Model file for the job. Use its own axes, mm. A direction names the side the tool comes from. Round coordinates to 2 decimals unless told otherwise and drop trailing zeros. Order: outer loops, then holes, each group sorted by start corner. A loop starts at its lowest first (then second) coordinate and runs counter-clockwise, first axis right, second up. Notation, with made-up numbers: M 25.5,-34 L 48.5,-34 A18 cw 48.5,-20 Z; hole C 55.5,53 d1. An arc over 180 degrees is marked long. Return JSON: item names as keys, results as strings. Group by question number.
Item 1: Pull direction X, two halves, no side cores. Call faces 5 (the face through (-5.5, -2, 0)), 6 (the face through (19, -13, 25)), 7 (the face through (42.5, -2, 0)): pulls with the +X half, pulls with the -X half, needs draft (parallel to the pull), parting line crosses it, or undercut.
Item 2: Slice it at C-C on x = 40.5. Write the cut outline in (y, z), then the cut area to 3 significant figures.
Item 3: Probe line 1 along Y through (x, z) = (50.5, 10); line 2 along X through (y, z) = (7.5, 2.5) (3 decimals); line 3 along Y through (x, z) = (-7, -16.5). List the from-to ranges inside material, lowest first.
Item 4: Slice it at A-A on z = -5. Write the cut outline in (x, y), then the cut area to 3 significant figures.
Item 5: Pin check, flat tips, straight feed: pin 1 Ø8 at (x, z) = (4, -3.5) entering from +Y; pin 2 Ø8 at (x, y) = (-1.5, 6.5) entering from -Z; pin 3 Ø1.5 at (x, z) = (-5, -13) entering from +Y. Stop position of each tip, or through.
Item 6: Slice it at B-B on y = 3. Write the cut outline in (x, z), then the cut area to 3 significant figures.
Item 7: Which spindle directions (+Z, -Z, +X, -X, +Y, -Y) get a long thin tool onto all of the face, cutting with end or side? Do faces 1 (the face through (-2, 0, -10)), 2 (the face through (-15, -19, 0)), 3 (the face through (39, 0, -10)), 4 (the face through (39, 0, 10)). Say none if no direction does.
Item 8: Slice it at D-D on z = -19.5. Write the cut outline in (x, y).
from build123d import *

# Parameters (mm, degrees)
EXTRUDE_1_DEPTH = 25
EXTRUDE_2_DEPTH = 10


with BuildPart() as part:
    # Sketch 1 → Extrude 1 (new, symmetric)
    with BuildSketch(Plane.XY):
        Polygon((18.5, 5), (18.5, 30), (3.083333333, 5), align=None)
        Polygon((3.083333333, 5), (-5.5, -8.918918919), (-5.5, -30), (18.5, -30), (18.5, 5), align=None)
        Polygon((-11.716666667, -19), (-18.5, -19), (-18.5, -30), (-5.5, -30), (-5.5, -8.918918919), align=None)
    extrude_1 = extrude(amount=EXTRUDE_1_DEPTH, both=True)

    # Sketch 1_3 → Extrude 2 (add, symmetric)
    with BuildSketch(Plane.XY):
        Polygon((-5.5, 5), (-5.5, -8.918918919), (3.083333333, 5), align=None)
    extrude_2 = extrude(amount=EXTRUDE_2_DEPTH, both=True)

    # Mirror 1: Extrude 1, Extrude 2 across plane
    add(extrude_1.mirror(Plane(origin=(18.5, 0, -25), x_dir=(0, 0, 1), z_dir=(1, 0, 0))))
    add(extrude_2.mirror(Plane(origin=(18.5, 0, -25), x_dir=(0, 0, 1), z_dir=(1, 0, 0))))


solid = part.part
Output values:
{
 "1": {"face 5": "pulls with the -X half", "face 6": "needs draft", "face 7": "pulls with the +X half"},
 "2": {"outline": "M -30,-25 L -5.68,-25 L -5.68,-10 L 5,-10 L 5,10 L -5.68,10 L -5.68,25 L -30,25 Z", "area": "1,430 mm²"},
 "3": {"line 1": "-30 to -19", "line 2": "4.625 to 32.375", "line 3": "-30 to -11.35"},
 "4": {"outline": "M -18.5,-30 L 55.5,-30 L 55.5,-19 L 48.72,-19 L 42.5,-8.92 L 42.5,5 L 33.92,5 L 18.5,30 L 3.08,5 L -5.5,5 L -5.5,-8.92 L -11.72,-19 L -18.5,-19 Z", "area": "2,410 mm²"},
 "5": {"pin 1": "y = 12.97", "pin 2": "z = -10", "pin 3": "y = -6.89"},
 "6": {"outline": "M -5.5,-10 L 1.85,-10 L 1.85,-25 L 35.15,-25 L 35.15,-10 L 42.5,-10 L 42.5,10 L 35.15,10 L 35.15,25 L 1.85,25 L 1.85,10 L -5.5,10 Z", "area": "1,960 mm²"},
 "7": {"face 1": "-Z, -X, +Y", "face 2": "+Z, -Z, -X, +Y", "face 3": "-Z, +X, +Y", "face 4": "+Z, +X, +Y"},
 "8": {"outline": "M -18.5,-30 L 55.5,-30 L 55.5,-19 L 48.72,-19 L 18.5,30 L -11.72,-19 L -18.5,-19 Z"}
}
